```python
from build123d import *

# Parameters (mm, degrees)
SKETCH_1_W          = 50
SKETCH_1_H          = 20
EXTRUDE_1_DEPTH     = 10
FILLET_1_R          = 2
SKETCH_2_R          = 4
CUT_EXTRUDE_1_DEPTH = 5


with BuildPart() as part:
    # 草图1 → 凸台-拉伸1 (new body)
    with BuildSketch(Plane.XY):
        with Locations((-10.973154362, 5.642841264)):
            Rectangle(SKETCH_1_W, SKETCH_1_H)
    extrude(amount=EXTRUDE_1_DEPTH)

    # 圆角1
    fillet_1_edges = [part.edges().sort_by_distance(p)[0] for p in [
        (14.026845638, 5.642841264, 10),
        (-10.973154362, 15.642841264, 10),
        (-35.973154362, 5.642841264, 10),
        (-10.973154362, -4.357158736, 10),
    ]]
    fillet(fillet_1_edges, radius=FILLET_1_R)

    # 草图2 → 切除-拉伸1 (cut)
    with BuildSketch(Plane(origin=(0, 0, 0), x_dir=(-1, 0, 0), z_dir=(0, 0, -1))):
        with Locations((10.973154362, 5.642841264)):
            Circle(SKETCH_2_R)
    extrude(amount=-CUT_EXTRUDE_1_DEPTH, mode=Mode.SUBTRACT)


solid = part.part
```
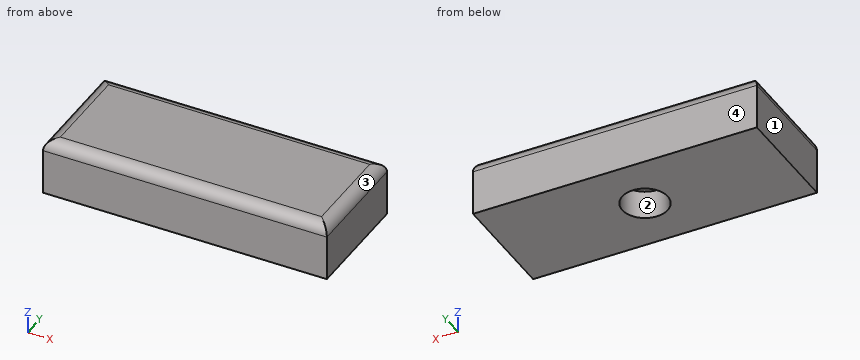
The model under review builds one solid part; all positions refer to its coordinate system, in mm. Face numbers are marked on the shaded views. Round coordinates to 2 decimals unless told otherwise and drop trailing zeros. Write each loop counter-clockwise with the first axis right and the second up, starting at its lowest first coordinate (ties: lowest second). Pieces come first, ordered by that corner, then holes. Notation, with made-up numbers: (64.5, 13) -> (80.5, 13) arc R27 cw to (80.5, 38) -> close; hole circle Ø11 at (37, -5). An arc over 180 degrees is marked (long way). Use CSV: the item, a comma, the result in double quotes.
Q1. Mouldability with a two-part tool opening along X and no side actions: class the marked faces 1, 2, 3 and 4 as released by +X, released by -X, zero draft, split by the parting line, or undercut.
Checks:
face 1,"released by -X"
face 2,"undercut"
face 3,"released by +X"
face 4,"zero draft"
Q2. To check wall thickness, follow probe 1 along Y at (x, z) = (-14, 2.75); probe 2 along Y at (x, z) = (-8.5, 1.5); probe 3 along X at (y, z) = (4.25, 9.25). State the ranges of each line that lie inside material, in increasing order. Write a range as [from, to].
Checks:
probe 1,"[-4.36, 3.03], [8.26, 15.64]"
probe 2,"[-4.36, 2.5], [8.79, 15.64]"
probe 3,"[-35.53, 13.59]"
Q3. Consider section A-A (z = 1). Give the boundary of the cut face in (x, y).
Checks:
outline,"(-35.97, -4.36) -> (14.03, -4.36) -> (14.03, 15.64) -> (-35.97, 15.64) -> close; hole circle Ø8 at (-10.97, 5.64)"
Q4. Consider section B-B (x = -9.5). Give the boundary of the cut face in (y, z), then the cut area to 3 significant figures.
Checks:
outline,"(-4.36, 0) -> (1.92, 0) -> (1.92, 5) -> (9.36, 5) -> (9.36, 0) -> (15.64, 0) -> (15.64, 8) arc R2 ccw to (13.64, 10) -> (-2.36, 10) arc R2 ccw to (-4.36, 8) -> close"
area,"161 mm²"
Q5. Consider section C-C (y = 7.75). Give the boundary of the cut face in (x, z).
Checks:
outline,"(-35.97, 0) -> (-14.37, 0) -> (-14.37, 5) -> (-7.57, 5) -> (-7.57, 0) -> (14.03, 0) -> (14.03, 8) arc R2 ccw to (12.03, 10) -> (-33.97, 10) arc R2 ccw to (-35.97, 8) -> close"
Q6. For pin 1 Ø2.5 at (x, y) = (-13, 5.5) entering from -Z, flat-tipped, find the tip position at first contact; note if it passes through.
Checks:
pin 1,"z = 5"
